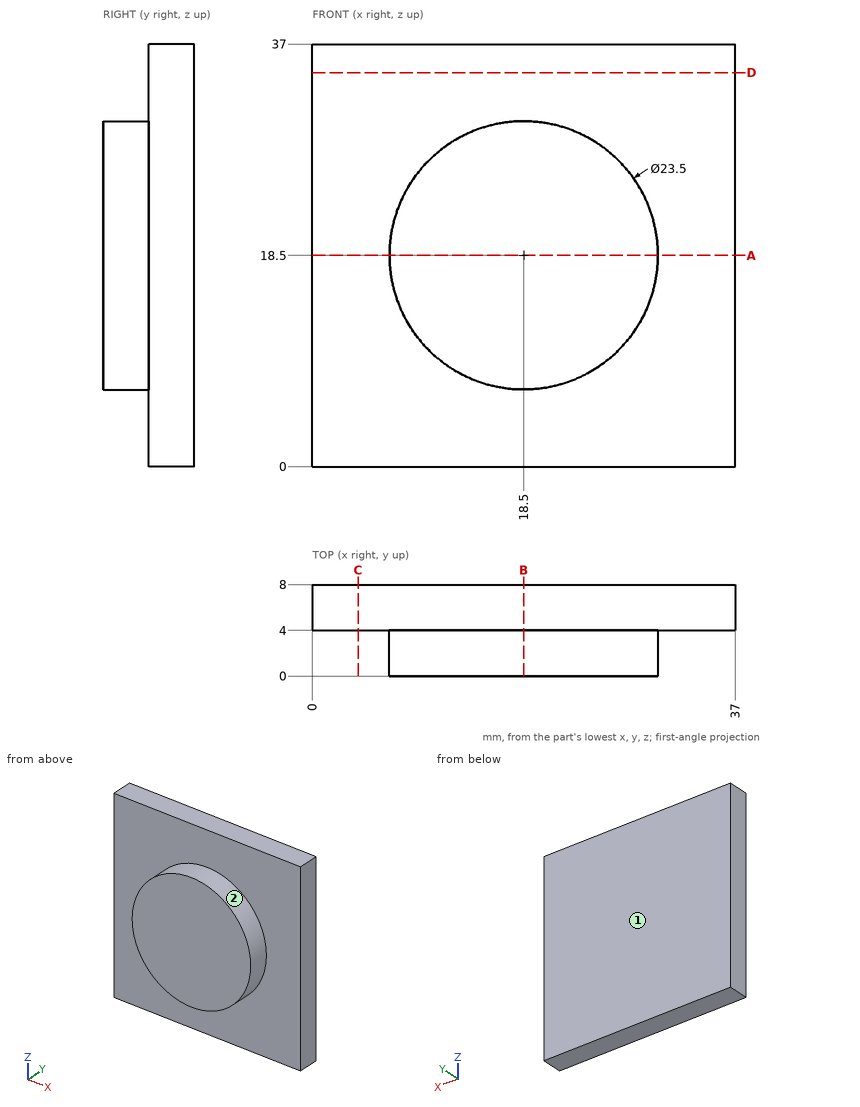
Input: dimensioned drawing with shaded views. Units: mm. Origin: part minimum x, y, z. A direction names the side the tool comes from. Round coordinates to 2 decimals unless told otherwise and drop trailing zeros. Loops run counter-clockwise (first coordinate to the right, second up) from the corner with the lowest first, then second, coordinate; pieces in that order, holes last. Notation, with made-up numbers: M 61.5,-7 L 72.5,-7 A36 ccw 72.5,29 Z; hole C 66,85 d7. An arc over 180 degrees is marked long. Answer in a Markdown table with one row per item. Add a question column.
1. Set-up query: the marked faces 1 and 2. Return all of +Z, -Z, +X, -X, +Y, -Y with unobstructed straight access to the full face (end or side cutting, diameter ignored); none if empty.
2. Section C-C (x = 4). Output: boundary loops of the cut face in (y, z), and give its area (3 significant figures).
3. Section D-D (z = 34.5). Output: boundary loops of the cut face in (x, y).
4. Section A-A (z = 18.5). Output: boundary loops of the cut face in (x, y).
5. Section B-B (x = 18.5). Output: boundary loops of the cut face in (y, z).
6. Ray query, probe 1 along Y at (x, z) = (29, 26); probe 2 along Z at (x, y) = (16, 2); probe 3 along X at (y, z) = (3.75, 17.5). Return the intervals inside material, ascending.
Values follow:
| question | item | result |
|---|---|---|
| 1 | face 1 | +Z, -Z, +X, -X, +Y |
| 1 | face 2 | -Y |
| 2 | outline | M 4,0 L 8,0 L 8,37 L 4,37 Z |
| 2 | area | 148 mm^2 |
| 3 | outline | M 0,4 L 37,4 L 37,8 L 0,8 Z |
| 4 | outline | M 0,4 L 6.75,4 L 6.75,0 L 30.25,0 L 30.25,4 L 37,4 L 37,8 L 0,8 Z |
| 5 | outline | M 0,6.75 L 4,6.75 L 4,0 L 8,0 L 8,37 L 4,37 L 4,30.25 L 0,30.25 Z |
| 6 | probe 1 | 4 to 8 |
| 6 | probe 2 | 7.02 to 29.98 |
| 6 | probe 3 | 6.79 to 30.21 |
